Read the model definition and answer for the solid it produces. Units are mm, in the model's axes. Face numbers are marked on the shaded views. Give positions to 0.01 mm unless a question says otherwise; leave off trailing zeros. Order: outer loops, then holes, each group sorted by start corner. A loop starts at its lowest first (then second) coordinate and runs counter-clockwise, first axis right, second up. Notation, with made-up numbers: (-11.75, 22) -> (36.25, 22) arc R13 cw to (36.25, 27) -> close; hole circle Ø1 at (19, -30). An arc over 180 degrees is marked (long way). Use one line per item in the form item = value.
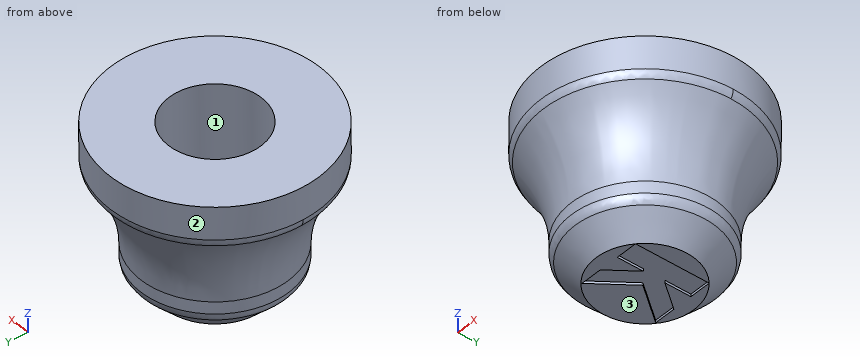
```python
from build123d import *

# Parameters (mm, degrees)
ESBO_O1_R                = 6
RESSALTO_EXTRUS_O1_DEPTH = 13
CORTE_EXTRUS_O1_DEPTH    = 12
ESBO_O3_R                = 3.75
CORTE_EXTRUS_O2_DEPTH    = 10
CHANFRO1_SIZE            = 2
ESBO_O4_R                = 8.5
ESBO_O4_R_2              = 3.75
RESSALTO_EXTRUS_O2_DEPTH = 3
FILETE1_R                = 10
FILETE3_R                = 1
CORTE_EXTRUS_O3_DEPTH    = 0.2


with BuildPart() as part:
    # Esboço1 → Ressalto-extrusão1 (new body)
    with BuildSketch(Plane.XY):
        with Locations(Location((0, 0, 0), (0, 0, 180))):
            Circle(ESBO_O1_R)
    extrude(amount=RESSALTO_EXTRUS_O1_DEPTH)

    # Esboço2 → Corte-extrusão1 (cut)
    with BuildSketch(Plane.XY.offset(13)):
        with BuildLine():
            Line((2.683281573, 1.45), (-2.683281573, 1.45))
            ThreePointArc((-2.683281573, 1.45), (-0.747827254, -2.956899457), (3.05, 0))
            ThreePointArc((3.05, 0), (2.956899457, 0.747827254), (2.683281573, 1.45))
        make_face()
    extrude(amount=-CORTE_EXTRUS_O1_DEPTH, mode=Mode.SUBTRACT)

    # Esboço3 → Corte-extrusão2 (cut)
    with BuildSketch(Plane.XY.offset(13)):
        Circle(ESBO_O3_R)
    extrude(amount=-CORTE_EXTRUS_O2_DEPTH, mode=Mode.SUBTRACT)

    # Chanfro1
    chanfro1_edges = [part.edges().sort_by_distance(p)[0] for p in [
        (6, 0, 0),
    ]]
    chamfer(chanfro1_edges, length=CHANFRO1_SIZE)

    # Esboço4 → Ressalto-extrusão2 (add)
    with BuildSketch(Plane.XY.offset(13)):
        Circle(ESBO_O4_R)
        Circle(ESBO_O4_R_2, mode=Mode.SUBTRACT)
    extrude(amount=-RESSALTO_EXTRUS_O2_DEPTH)

    # Filete1
    # the kernel refuses this fillet: 10 mm, written as the material it adds along each edge
    with BuildSketch(Plane(origin=(0, 0, 10), x_dir=(-1, 0, 0), z_dir=(0, -1, 0))) as filete1_piece_1:
        with BuildLine():
            CenterArc((16, 6.614378278), FILETE1_R, 180, 41.409622109)
            Line((8.5, 0), (6, 0))
            Line((6, 0), (6, 6.614378278))
        make_face()
    revolve(axis=Axis((0, 0, 10), (0, 0, -1)))

    # Filete3
    filete3_edges = [part.edges().sort_by_distance(p)[0] for p in [
        (6, 0, 2),
        (0, 8.5, 10),
    ]]
    fillet(filete3_edges, radius=FILETE3_R)

    # Esboço5 → Corte-extrusão3 (cut)
    with BuildSketch(Plane(origin=(0, 0, 0), x_dir=(-1, 0, 0), z_dir=(0, 0, -1))):
        Polygon((-2.631008166, 3.012938106), (-2.631008166, -3.012938106), (-0.875588874, -3.012938106), (-0.875588874, -0.877709646), (0.761455767, -3.012938106), (2.51687506, -3.012938106), (0.206904827, 0), (2.51687506, 3.012938106), (0.761455767, 3.012938106), (-0.875588874, 0.877709646), (-0.875588874, 3.012938106), align=None)
    extrude(amount=-CORTE_EXTRUS_O3_DEPTH, mode=Mode.SUBTRACT)


solid = part.part
```
Item 1: Straight lines are drawn through the part: L1, parallel to X at y = 0, z = 2.45; L2, parallel to Y at x = 0, z = 9; L3, parallel to X at y = 1, z = 3.75. For each, find the intervals that lie inside material, in ascending order. Write a range as from..to.
Checks:
L1 = -6..-3.05, 3.05..6
L2 = -7.72..-3.75, 3.75..7.72
L3 = -5.92..-3.61, 3.61..5.92
Item 2: The part is cut by section A-A on z = 4. Give the vertices of the cut face in (x, y), and give its area (3 significant figures).
Checks:
outline = circle Ø12.04 at (0, 0); hole circle Ø7.5 at (0, 0)
area = 69.6 mm²
Item 3: Given pin 1 Ø3 at (y, z) = (-4.5, 3) entering from -X; pin 2 Ø1 at (x, z) = (-6, 6.5) entering from +Y; pin 3 Ø2 at (x, y) = (-0.5, 1) entering from +Z, each flat-ended and moving along its own axis, determine where each tip first touches the part or whether it passes through.
Checks:
pin_1 = -5.2
pin_2 = 3.52
pin_3 = 3
Item 4: Determine the mould class of the marked faces 1, 2 and 3 for opening direction X: +X half, -X half, draft (parallel to the pull), parting line (faces both ways), or undercut.
Checks:
face_1 = undercut
face_2 = parting line
face_3 = draft
